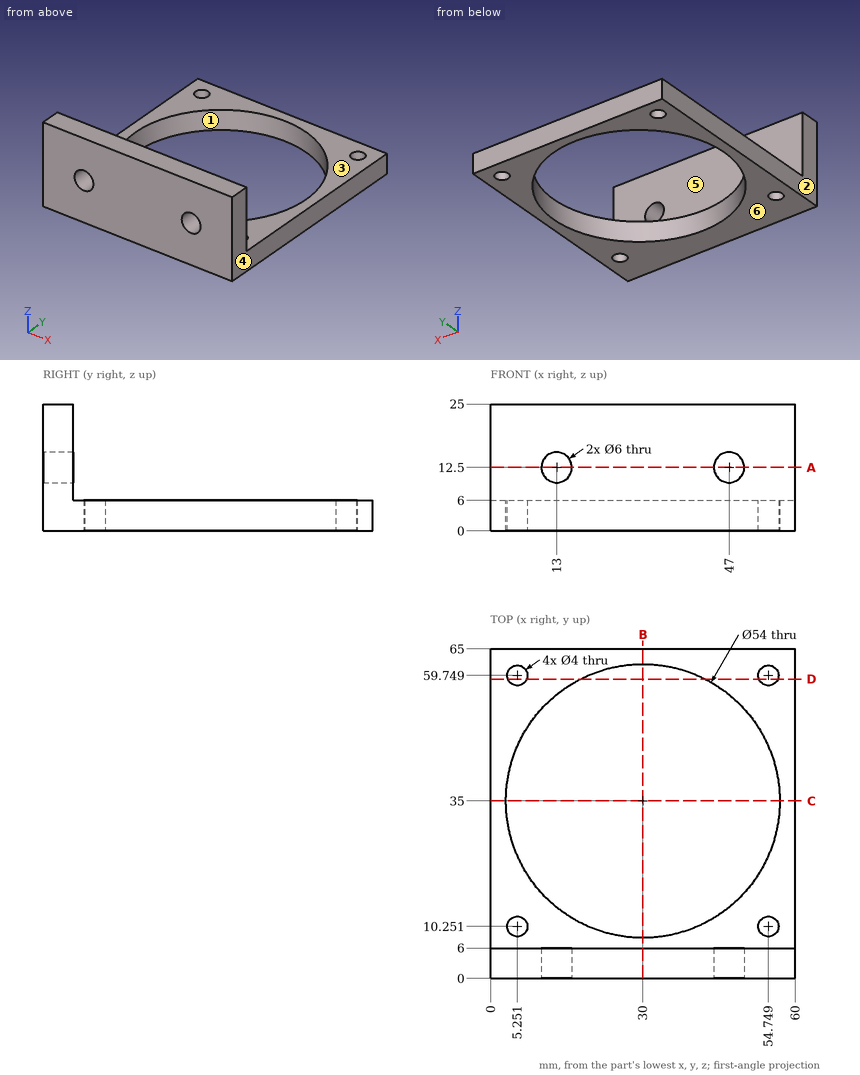
Source: three-view drawing plus pictorial views. Frame: mm from the lowest corner of the part. A direction names the side the tool comes from. Round coordinates to 2 decimals unless told otherwise and drop trailing zeros. Loops run counter-clockwise (first coordinate to the right, second up) from the corner with the lowest first, then second, coordinate; pieces in that order, holes last. Notation, with made-up numbers: (30, 24) -> (37, 24) arc R25 cw to (37, 62) -> close; hole circle Ø3 at (53.25, -18). An arc over 180 degrees is marked (long way). Use one line per item in the form item = value.
Item 1: Cut plane D-D on y = 59. Output: boundary loops of the cut face in (x, z).
Evaluation:
outline = (0, 0) -> (3.4, 0) -> (3.4, 6) -> (0, 6) -> close; (7.11, 0) -> (17.63, 0) -> (17.63, 6) -> (7.11, 6) -> close; (42.37, 0) -> (52.89, 0) -> (52.89, 6) -> (42.37, 6) -> close; (56.6, 0) -> (60, 0) -> (60, 6) -> (56.6, 6) -> close
Item 2: Cut plane C-C on y = 35. Output: boundary loops of the cut face in (x, z).
Evaluation:
outline = (0, 0) -> (3, 0) -> (3, 6) -> (0, 6) -> close; (57, 0) -> (60, 0) -> (60, 6) -> (57, 6) -> close
Item 3: Draft query along X for the marked faces 1, 2, 3 and 4. Return one class per face: released by +X, released by -X, zero draft, split by the parting line, or undercut.
Evaluation:
face_1 = undercut
face_2 = released by -X
face_3 = zero draft
face_4 = released by +X
Item 4: Cut plane A-A on z = 12.5. Output: boundary loops of the cut face in (x, y).
Evaluation:
outline = (0, 0) -> (10, 0) -> (10, 6) -> (0, 6) -> close; (16, 0) -> (44, 0) -> (44, 6) -> (16, 6) -> close; (50, 0) -> (60, 0) -> (60, 6) -> (50, 6) -> close
Item 5: Cut plane B-B on x = 30. Output: boundary loops of the cut face in (y, z), then the cut area to 3 significant figures.
Evaluation:
outline = (0, 0) -> (8, 0) -> (8, 6) -> (6, 6) -> (6, 25) -> (0, 25) -> close; (62, 0) -> (65, 0) -> (65, 6) -> (62, 6) -> close
area = 180 mm2
Item 6: Material intervals for probe 1 along X at (y, z) = (2.55, 12.5); probe 2 along Y at (x, z) = (30, 5.25); probe 3 along Z at (x, y) = (45, 61.5), sorted ascending.
Evaluation:
probe_1 = 0 to 10, 16 to 44, 50 to 60
probe_2 = 0 to 8, 62 to 65
probe_3 = 0 to 6
Item 7: Access query for the marked faces 5 and 6. Directions: +Z, -Z, +X, -X, +Y, -Y. A direction counts if a zero-diameter tool reaches every point of the face in a straight line with its end or side. Return the directions, or none.
Evaluation:
face_5 = +Z, +X, -X, +Y
face_6 = -Z, +X, -X, +Y, -Y
Item 8: Contact query for flat-ended pins moving along their axis: pin 1 Ø5 at (x, y) = (54.75, 59.75) entering from -Z; pin 2 Ø2 at (x, y) = (7.5, 16) entering from +Z. Output: stop coordinate, or through.
Evaluation:
pin_1 = 0
pin_2 = 6
